```python
from build123d import *

# Parameters (mm, degrees)
SKETCH_1_W            = 90
SKETCH_1_H            = 120
SKETCH_1_R            = 2
SKETCH_1_R_2          = 1.6
EXTRUDE_1_DEPTH       = 5
FILLET_1_R            = 8
F_3_2_PCD16_R         = 1.6
CUT_EXTRUDE_3_2_DEPTH = 10
F_6_PCD16_R           = 3
CUT_EXTRUDE_6_1_DEPTH = 1


with BuildPart() as part:
    # 草图1 → 凸台-拉伸1 (new body)
    with BuildSketch(Plane.XY):
        with Locations((45, -60)):
            Rectangle(SKETCH_1_W, SKETCH_1_H)
        with Locations((79, -45)):
            Circle(SKETCH_1_R, mode=Mode.SUBTRACT)
        with Locations((79, -75)):
            Circle(SKETCH_1_R, mode=Mode.SUBTRACT)
        with Locations((49, -45)):
            Circle(SKETCH_1_R, mode=Mode.SUBTRACT)
        with Locations((49, -75)):
            Circle(SKETCH_1_R, mode=Mode.SUBTRACT)
        with Locations((85, -102.5)):
            Circle(SKETCH_1_R_2, mode=Mode.SUBTRACT)
        with Locations((75, -102.5)):
            Circle(SKETCH_1_R_2, mode=Mode.SUBTRACT)
        with Locations((65, -102.5)):
            Circle(SKETCH_1_R_2, mode=Mode.SUBTRACT)
        with Locations((55, -102.5)):
            Circle(SKETCH_1_R_2, mode=Mode.SUBTRACT)
        with Locations((45, -102.5)):
            Circle(SKETCH_1_R_2, mode=Mode.SUBTRACT)
        with Locations((85, -17.5)):
            Circle(SKETCH_1_R_2, mode=Mode.SUBTRACT)
        with Locations((75, -17.5)):
            Circle(SKETCH_1_R_2, mode=Mode.SUBTRACT)
        with Locations((65, -17.5)):
            Circle(SKETCH_1_R_2, mode=Mode.SUBTRACT)
        with Locations((55, -17.5)):
            Circle(SKETCH_1_R_2, mode=Mode.SUBTRACT)
        with Locations((45, -17.5)):
            Circle(SKETCH_1_R_2, mode=Mode.SUBTRACT)
        with Locations((35, -102.5)):
            Circle(SKETCH_1_R_2, mode=Mode.SUBTRACT)
        with Locations((25, -102.5)):
            Circle(SKETCH_1_R_2, mode=Mode.SUBTRACT)
        with Locations((15, -102.5)):
            Circle(SKETCH_1_R_2, mode=Mode.SUBTRACT)
        with Locations((35, -17.5)):
            Circle(SKETCH_1_R_2, mode=Mode.SUBTRACT)
        with Locations((25, -17.5)):
            Circle(SKETCH_1_R_2, mode=Mode.SUBTRACT)
        with Locations((15, -17.5)):
            Circle(SKETCH_1_R_2, mode=Mode.SUBTRACT)
        with Locations((8, -102.5)):
            Circle(SKETCH_1_R_2, mode=Mode.SUBTRACT)
        with Locations((8, -17.5)):
            Circle(SKETCH_1_R_2, mode=Mode.SUBTRACT)
    extrude(amount=EXTRUDE_1_DEPTH)

    # 圆角1
    fillet_1_edges = [part.edges().sort_by_distance(p)[0] for p in [
        (0, 0, 2.5),
        (90, 0, 2.5),
        (90, -120, 2.5),
        (0, -120, 2.5),
    ]]
    fillet(fillet_1_edges, radius=FILLET_1_R)

    # 内圈四孔_Ø3.2_PCD16 → 内圈四孔_通孔_Ø3.2 (cut)
    with BuildSketch(Plane(origin=(0, 0, 0), x_dir=(-1, 0, 0), z_dir=(0, 0, -1))):
        with Locations((-46.156854249, -54.343145751)):
            Circle(F_3_2_PCD16_R)
        with Locations((-34.843145751, -54.343145751)):
            Circle(F_3_2_PCD16_R)
        with Locations((-34.843145751, -65.656854249)):
            Circle(F_3_2_PCD16_R)
        with Locations((-46.156854249, -65.656854249)):
            Circle(F_3_2_PCD16_R)
    extrude(amount=-CUT_EXTRUDE_3_2_DEPTH, mode=Mode.SUBTRACT)

    # 内圈沉孔_Ø6_PCD16 → 内圈四孔_沉孔_Ø6深1 (cut)
    with BuildSketch(Plane(origin=(0, 0, 0), x_dir=(-1, 0, 0), z_dir=(0, 0, -1))):
        with Locations((-46.156854249, -54.343145751)):
            Circle(F_6_PCD16_R)
        with Locations((-34.843145751, -54.343145751)):
            Circle(F_6_PCD16_R)
        with Locations((-34.843145751, -65.656854249)):
            Circle(F_6_PCD16_R)
        with Locations((-46.156854249, -65.656854249)):
            Circle(F_6_PCD16_R)
    extrude(amount=-CUT_EXTRUDE_6_1_DEPTH, mode=Mode.SUBTRACT)


solid = part.part
```
Part model, mm, in its own coordinate system. A direction names the side the tool comes from. Round coordinates to 2 decimals unless told otherwise and drop trailing zeros. Write each loop counter-clockwise with the first axis right and the second up, starting at its lowest first coordinate (ties: lowest second). Pieces come first, ordered by that corner, then holes.
Item 1: Cut at D-D, the plane y = -102.5. Count the separate pieces of the cut face and the enclosed holes in it, plus the area to 3 significant figures.
Results:
separate pieces: 10
enclosed holes: 0
area: 306 mm2
Item 2: Which spindle directions (+Z, -Z, +X, -X, +Y, -Y) get a long thin tool onto all of the face, cutting with end or side? Do faces 4 (the cylindrical face through (7.792, -15.914, 2.465)), 5 (the flat face through (45, -67, 1)). Say none if no direction does.
Results:
face 4: +Z, -Z
face 5: -Z
Item 3: Two-plate mould, pull along X, no slides. Class faces 1 (the cylindrical face through (66.526, -102.019, 2.465)), 2 (the cylindrical face through (2.281, -2.406, 2.535)), 3 (the cylindrical face through (87.594, -2.281, 2.535)): +X half, -X half, draft (parallel to the pull), parting line (faces both ways), or undercut.
Results:
face 1: undercut
face 2: -X half
face 3: +X half
Item 4: Drop flat-ended pins along their axis: pin 1 Ø5 at (x, y) = (45.5, -67) entering from -Z; pin 2 Ø5 at (x, y) = (46.16, -65.66) entering from -Z. Give the stop position or say it passes through.
Results:
pin 1: stops at z = 0
pin 2: stops at z = 1
Item 5: Probe L1, parallel to Y at x = 79, z = 4.35; L2, parallel to Y at x = 55, z = 1.8; L3, parallel to Y at x = 35, z = 4.05. List the from-to ranges inside material, lowest first.
Results:
L1: y = -120 to -77, -73 to -47, -43 to 0
L2: y = -120 to -104.1, -100.9 to -19.1, -15.9 to 0
L3: y = -120 to -104.1, -100.9 to -67.25, -64.06 to -55.94, -52.75 to -19.1, -15.9 to 0
Item 6: Cut at B-B, the plane y = -75. Give the cut face in (x, z).
Results:
outline: (0, 0) - (47, 0) - (47, 5) - (0, 5) - close; (51, 0) - (77, 0) - (77, 5) - (51, 5) - close; (81, 0) - (90, 0) - (90, 5) - (81, 5) - close
Item 7: Cut at A-A, the plane x = 15. Give the cut face in (y, z), plus the area to 3 significant figures.
Results:
outline: (-120, 0) - (-104.1, 0) - (-104.1, 5) - (-120, 5) - close; (-100.9, 0) - (-19.1, 0) - (-19.1, 5) - (-100.9, 5) - close; (-15.9, 0) - (0, 0) - (0, 5) - (-15.9, 5) - close
area: 568 mm2
Item 8: Cut at C-C, the plane x = 35. Give the cut face in (y, z).
Results:
outline: (-120, 0) - (-104.1, 0) - (-104.1, 5) - (-120, 5) - close; (-100.9, 0) - (-68.65, 0) - (-68.65, 1) - (-67.25, 1) - (-67.25, 5) - (-100.9, 5) - close; (-64.06, 1) - (-62.66, 1) - (-62.66, 0) - (-57.34, 0) - (-57.34, 1) - (-55.94, 1) - (-55.94, 5) - (-64.06, 5) - close; (-52.75, 1) - (-51.35, 1) - (-51.35, 0) - (-19.1, 0) - (-19.1, 5) - (-52.75, 5) - close; (-15.9, 0) - (0, 0) - (0, 5) - (-15.9, 5) - close
